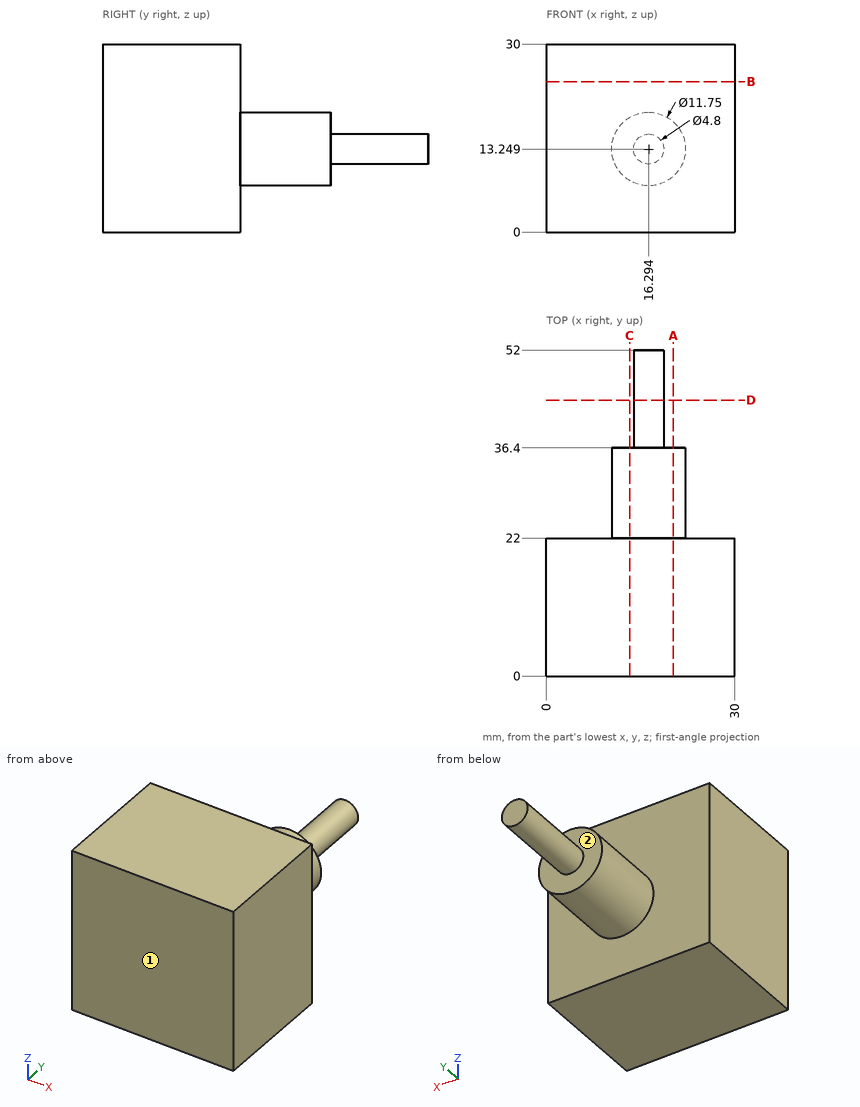
Study the drawing (mm; zero at the part's minimum x, y, z) and answer. A direction names the side the tool comes from. Coordinates: 2 decimals unless noted, no trailing zeros. Write each loop counter-clockwise with the first axis right and the second up, starting at its lowest first coordinate (ties: lowest second). Pieces come first, ordered by that corner, then holes. Notation, with made-up numbers: M -29,-35.5 L 20,-35.5 A38 ccw 20,2.5 Z; hole C 31.5,-27.75 d2. An arc over 180 degrees is marked long. Use a Markdown table: item, result. Add a question column.
1. Given P1, Ø10, axis at x = 10, y = 45.5, coming from the -Z side; P2, Ø6, axis at y = 37, z = 18, coming from the +X side; P3, Ø1.5, axis at x = 25, z = 26, coming from the +Y side, each flat-ended and moving along its own axis, determine where each tip first touches the part or whether it passes through.
2. Section B-B (z = 24) is taken. Give the vertices of the cut face in (x, y).
3. Section D-D (y = 44) is taken. Give the vertices of the cut face in (x, z) (1 decimal).
4. Section A-A (x = 20.25) is taken. Give the vertices of the cut face in (y, z) (1 decimal).
5. Which of the six approach directions +Z, -Z, +X, -X, +Y, -Y give full straight-line access (tool end or side, diameter ignored) to the marked faces 1 and 2?
6. Straight lines are drawn through the part: line 1 along Y through (x, z) = (21, 22.75); line 2 along X through (y, z) = (24, 11.5) (1 decimal); line 3 along X through (y, z) = (43, 14) (1 decimal). For each, find the intervals that lie inside material, in ascending order. Write a range as [from, to].
7. Section C-C (x = 13.25) is taken. Give the vertices of the cut face in (y, z), plus the area to 3 significant figures.
Data:
| question | item | result |
|---|---|---|
| 1 | P1 | stops at z = 11.23 |
| 1 | P2 | stops at x = 21.88 |
| 1 | P3 | stops at y = 22 |
| 2 | outline | M 0,0 L 30,0 L 30,22 L 0,22 Z |
| 3 | outline | C 16.3,13.2 d4.8 |
| 4 | outline | M 0,0 L 22,0 L 22,8.9 L 36.4,8.9 L 36.4,17.6 L 22,17.6 L 22,30 L 0,30 Z |
| 5 | face 1 | +Z, -Z, +X, -X, -Y |
| 5 | face 2 | +Y |
| 6 | line 1 | y = [0, 22] |
| 6 | line 2 | x = [10.7, 21.9] |
| 6 | line 3 | x = [14, 18.6] |
| 7 | outline | M 0,0 L 22,0 L 22,8.22 L 36.4,8.22 L 36.4,18.27 L 22,18.27 L 22,30 L 0,30 Z |
| 7 | area | 805 mm2 |
